Autodesk Inventor part; units mm, degrees
ref_plane "Work Plane1" through (-19.2723, 0, 0) normal (0, -0.866, -0.5) x (1, 0, 0)
ref_plane "YZ Plane" through (0, 0, 0) normal (1, 0, 0) x (0, 1, 0)
ref_plane "XZ Plane" through (0, 0, 0) normal (0, 1, 0) x (-1, 0, 0)
sketch "Эскиз1" plane through (0, 0, 0) normal (1, 0, 0) x (0, 1, 0)
  line L0 (-9.815, 0) -> (-4.9075, 8.5)
  line L1 (-4.9075, 8.5) -> (4.9075, 8.5)
  line L2 (4.9075, 8.5) -> (9.815, 0)
  line L3 (9.815, 0) -> (4.9075, -8.5)
  line L4 (4.9075, -8.5) -> (-4.9075, -8.5)
  line L5 (-4.9075, -8.5) -> (-9.815, 0)
  point P0 (0, 0)
  point P1 (0, 0)
  dimension "d0" = 19.6299
extrude "Базовый элемент" add sketch "Эскиз1" along normal blind 8
sketch "Эскиз2" plane through (0, 0, 0) normal (0, 0, 1) x (1, 0, 0)
  line L0 (0, 4.9075) -> (0, 9.815)
  line L1 (0, 9.815) -> (8, 9.815)
  line L2 (8, 4.9075) -> (8, 9.815)
  line L3 (-1.6, 0) -> (9.6, 0)
  line L4 (1.2499, 9.815) -> (0, 7.65)
  line L5 (6.7501, 9.815) -> (8, 7.65)
  dimension "d3" = 30
  dimension "d4" = 30
  dimension "d5" = 15.3
  dimension "d6" = 15.3
revolve "Фаска1" cut sketch "Эскиз2" angle 360 about axis through (-10, 0, 0) along (1, 0, 0)
sketch "Эскиз3" plane through (8, 0, 0) normal (1, 0, 0) x (0, 0, -1)
  arc A0 (-0.625, -1.0825) -> (0.625, -1.0825) centre (0, 0) ccw
hole "Резьба" at (8, 0, 0) direction (-1, 0, 0) diameter 8.376 end through all
chamfer "Фаска2" distance 0.8119 angle 30 1 edges at (8, 0, 4.188) measured on face at (8, 6.4117, -0.7785)
chamfer "Фаска3" distance 0.8119 angle 30 1 edges at (0, 0, 4.188) measured on face at (0, 6.4117, -0.7785)
ref_plane "Work Plane1" through (-19.2723, 0, 0) normal (0, -0.866, -0.5) x (1, 0, 0)
equation "\"d0\" = 1.1547 * SW"
equation "\"d1\" = KOH"
equation "\"d3\" = ANG1"
equation "\"d4\" = ANG2"
equation "\"d5\" = SW0"
equation "\"d6\" = SW01"
equation "\"d8\" = -0.5 * GD1 + 0.5 * NND"
equation "\"d40\" = -0.5 * GD1 + 0.5 * NND"
equation "\"d10\" = -0.5 * GD1 + 0.5 * NND"
equation "\"d41\" = -0.5 * GD1 + 0.5 * NND"
equation "\"ANG1\" = 30deg"
equation "\"ANG2\" = 30deg"
equation "\"KOH\" = 8"
equation "\"SW\" = 17"
equation "\"SW0\" = 15.3"
equation "\"SW01\" = SW0"
equation "\"GUL\" = 0.541266 * PTC"
equation "\"LADI\" = 16.15"
equation "\"TOA\" = 30deg"
equation "\"FAWI\" = 30deg"
equation "\"PTC\" = 1.5"
equation "\"E0\" = 1.155 * SW"
equation "\"GAL\" = 0.541266 * PTC"
properties part number "Гайка M10-6H ГОСТ 5915-70(1)" material "Сталь, мягкая"
The model under review builds one solid part; all positions refer to its coordinate system, in mm. Give positions to 0.01 mm unless a question says otherwise; leave off trailing zeros. Order: outer loops, then holes, each group sorted by start corner. A loop starts at its lowest first (then second) coordinate and runs counter-clockwise, first axis right, second up. Notation, with made-up numbers: (88.5, 59.25) - (111.5, 59.25) arc R28 ccw to (111.5, 90.25) - close; hole circle Ø6 at (75, -40). An arc over 180 degrees is marked (long way). Use CSV: the item, a comma, the result in double quotes. Start each with the question number.
Q1. We need section B-B, the plane x = 4.5. Write out the cut boundary in (y, z) (1 decimal), and give its area (3 significant figures).
Q2. The part is to be moulded in two halves that separate along Y. For faces 1 (the flat face through (0, 2, -5)), 2 (the cylindrical face through (3.951, -2.83, 3.087)), 3 (the conical face through (7.92, -7.78, -0.34)), 4 (the flat face through (3.951, 7.396, -4.19)), say which applies: +Y half, -Y half, draft (parallel to the pull), parting line (faces both ways), or undercut.
Q3. To check wall thickness, follow line 1 along Z through (x, y) = (5, 0); line 2 along X through (y, z) = (-7.75, 3.5); line 3 along Y through (x, z) = (5, -0.5). State the ranges of each line that lie inside material, in increasing order. Write a range as [from, to].
Q4. We need section A-A, the plane y = 0. Write out the cut boundary in (x, z).
Q5. Clearance check with flat-ended pins moving along their axes: pin 1 Ø6.5 at (y, z) = (0, 0) entering from -X; pin 2 Ø4 at (y, z) = (-7.5, 2.5) entering from +X; pin 3 Ø2 at (x, y) = (5, -7) entering from -Z; pin 4 Ø4 at (x, y) = (2.5, 7) entering from -Z. State where each tip first meets the part, or that it passes through.
Outcome:
1,outline,"(-9.8, 0) - (-4.9, -8.5) - (4.9, -8.5) - (9.8, 0) - (4.9, 8.5) - (-4.9, 8.5) - close; hole circle Ø8.4 at (0, 0)"
1,area,"195 mm^2"
2,face 1,"draft"
2,face 2,"undercut"
2,face 3,"parting line"
2,face 4,"+Y half"
3,line 1,"z = [-8.5, -4.19], [4.19, 8.5]"
3,line 2,"x = [0.49, 7.51]"
3,line 3,"y = [-9.53, -4.16], [4.16, 9.53]"
4,outline,"(0, -7.65) - (0.49, -8.5) - (7.51, -8.5) - (8, -7.65) - (8, -5) - (7.53, -4.19) - (0.47, -4.19) - (0, -5) - close; (0, 5) - (0.47, 4.19) - (7.53, 4.19) - (8, 5) - (8, 7.65) - (7.51, 8.5) - (0.49, 8.5) - (0, 7.65) - close"
5,pin 1,"passes through"
5,pin 2,"stops at x = 8"
5,pin 3,"stops at z = -6.61"
5,pin 4,"stops at z = -8.34"
